Check sheet for the modelled part. Datum: model origin and axes. Units: mm. Face numbers are marked on the shaded views. A direction names the side the tool comes from. Give positions to 0.01 mm unless a question says otherwise; leave off trailing zeros. Loops run counter-clockwise (first coordinate to the right, second up) from the corner with the lowest first, then second, coordinate; pieces in that order, holes last. Notation, with made-up numbers: M -9,68 L 11,68 A29 ccw 11,102 Z; hole C -0.75,-36 d3. An arc over 180 degrees is marked long. Put each result on its own line as item: value. Start each with the question number.
```python
from build123d import *

# Parameters (mm, degrees)
CYLINDER019_R          = 2.5
CYLINDER019_DEPTH      = 10
CYLINDER016_R          = 2.5
CYLINDER016_DEPTH      = 10
CYLINDER017_W          = 35
CYLINDER017_H          = 19
CYLINDER017_ANGLE      = 25
CYLINDER018_W          = 35
CYLINDER018_H          = 19
CYLINDER018_ANGLE      = 25
BOX028_W               = 19
BOX028_H               = 50
BOX028_DEPTH           = 4
BOX003_W               = 140
BOX003_H               = 162
BOX003_DEPTH           = 4
BOX003_ROLL_ANGLE      = 25.000043
BOX003_PLACEMENT_ANGLE = 180
BOX032_W               = 19
BOX032_H               = 29
BOX032_DEPTH           = 8
BOX032_PLACEMENT_ANGLE = 25


with BuildPart() as m4s003:
    # Cylinder019 → Cylinder019 (new body)
    with BuildSketch(Plane(origin=(177.5, 240.5, 0), x_dir=(1, 0, 0), z_dir=(0, 0, 1))):
        Circle(CYLINDER019_R)
    extrude(amount=CYLINDER019_DEPTH)


with BuildPart() as m4lowcut001:
    # Cylinder016 → Cylinder016 (new body)
    with BuildSketch(Plane(origin=(177.5, 252.5, 0), x_dir=(1, 0, 0), z_dir=(0, 0, 1))):
        Circle(CYLINDER016_R)
    extrude(amount=CYLINDER016_DEPTH)

    # Fusion010: union m4s003
    add(m4s003.part)


with BuildPart() as cylinder017:
    # Cylinder017 → Cylinder017 (revolve)
    with BuildSketch(Plane(origin=(187, 283, 4), x_dir=(0, -1, 0), z_dir=(0, 0, -1))):
        with Locations((17.5, 9.5)):
            Rectangle(CYLINDER017_W, CYLINDER017_H)
    revolve(axis=Axis((187, 283, 4), (-1, 0, 0)), revolution_arc=CYLINDER017_ANGLE)


with BuildPart() as bottom002:
    # Cylinder018 → Cylinder018 (revolve)
    with BuildSketch(Plane(origin=(187, 292.5, 4), x_dir=(0, -1, 0), z_dir=(0, 0, -1))):
        with Locations((17.5, 9.5)):
            Rectangle(CYLINDER018_W, CYLINDER018_H)
    revolve(axis=Axis((187, 292.5, 4), (-1, 0, 0)), revolution_arc=CYLINDER018_ANGLE)

    # Cut016: cut Cylinder017
    add(cylinder017.part, mode=Mode.SUBTRACT)


with BuildPart() as bottomright:
    # Box028 → Box028 (new body)
    with BuildSketch(Plane(origin=(168, 233.5, 4), x_dir=(1, 0, 0), z_dir=(0, 0, 1))):
        with Locations((9.5, 25)):
            Rectangle(BOX028_W, BOX028_H)
    extrude(amount=BOX028_DEPTH)

    # Fusion009: union bottom002
    add(bottom002.part)

    # Cut017: cut m4lowCut001
    add(m4lowcut001.part, mode=Mode.SUBTRACT)


with BuildPart() as bottomright_1:
    # Cut017 placement: moved
    add(bottomright.part.moved(Location((144, 0, 0))))


with BuildPart() as solar_panel002:
    # Box003 → Box003 (new body)
    with BuildSketch(Plane.XY):
        with Locations((70, 81)):
            Rectangle(BOX003_W, BOX003_H)
    extrude(amount=BOX003_DEPTH)


with BuildPart() as solar_panel002_1:
    # Box003 roll: moved
    add(solar_panel002.part.rotate(Axis((0, 0, 0), (1, 0, 0)), BOX003_ROLL_ANGLE))


with BuildPart() as solar_panel002_2:
    # Box003 placement: moved
    add(solar_panel002_1.part.moved(Location((321.5, 284, 8))).rotate(Axis((321.5, 284, 8), (0, 0, 1)), BOX003_PLACEMENT_ANGLE))


with BuildPart() as topright001:
    # Box032 → Box032 (new body)
    with BuildSketch(Plane.XY):
        with Locations((9.5, 14.5)):
            Rectangle(BOX032_W, BOX032_H)
    extrude(amount=BOX032_DEPTH)


with BuildPart() as topright001_1:
    # Box032 placement: moved
    add(topright001.part.moved(Location((312, 260.906, 18.73))).rotate(Axis((312, 260.906, 18.73), (-1, 0, 0)), BOX032_PLACEMENT_ANGLE))

    # Cut024: cut solar Panel002
    add(solar_panel002_2.part, mode=Mode.SUBTRACT)

    # Fusion028: union bottomRight
    add(bottomright_1.part)


solid = topright001_1.part
```
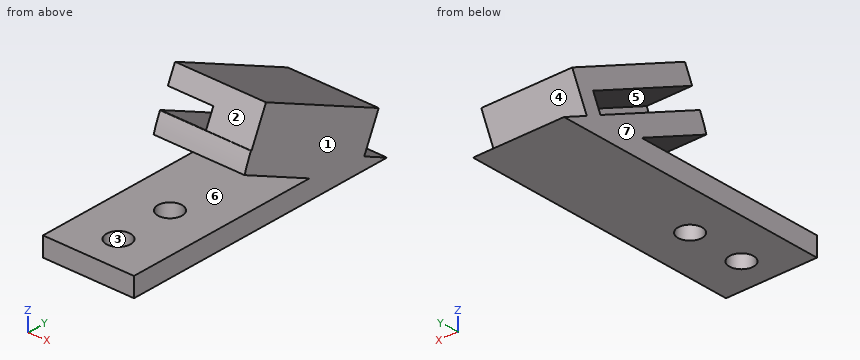
Q1. Access from +Z, -Z, +X, -X, +Y, -Y to the whole of each face (thin tool, end or side, straight path). Record for the marked faces 4, 5, 6 and 7.
Q2. Thickness scan on line 1 along X through (y, z) = (240.5, 5.35); line 2 along Z through (x, y) = (315.75, 268); line 3 along Z through (x, y) = (317, 271). Record the ranges inside material, lowest first. Write a range as [from, to].
Q3. Depth check by flat-ended pin: P1, Ø1.5, axis at x = 322.5, z = 16.5, coming from the -Y side; P2, Ø4, axis at x = 316, y = 247.5, coming from the +Z side; P3, Ø10, axis at x = 322, z = 20, coming from the -Y side. Enter the tip coordinate at first touch or a pass-through.
Q4. Mould release check, pull along X, two halves, no side actions. Record for the marked faces 1, 2 and 3: pulls with the +X half, pulls with the -X half, needs draft (parallel to the pull), parting line crosses it, or undercut.
Q5. Section check D-D, the plane z = 16.5. Record the cut outline in (x, y), then the cut area to 3 significant figures.
Q6. Section check B-B, the plane x = 319.75. Give the number of separate pieces and of enclosed holes in the cut face, then the cut area to 3 significant figures.
Q7. Section check A-A, the plane y = 240.5. Record the cut outline in (x, z), then the cut area to 3 significant figures.
Found:
1. face 4: +X, -X, +Y
1. face 5: -X
1. face 6: +X, -X, -Y
1. face 7: +Z, -Z, -X, +Y, -Y
2. line 1: x = [312, 319], [324, 331]
2. line 2: z = [4, 8], [10.99, 15.46], [19.87, 24.25]
2. line 3: z = [4, 8], [9.6, 14.06], [18.48, 22.85]
3. P1: stops at y = 259.53
3. P2: stops at z = 8
3. P3: stops at y = 259.29
4. face 1: pulls with the +X half
4. face 2: needs draft
4. face 3: undercut
5. outline: M 312,259.81 L 331,259.81 L 331,284.62 L 312,284.62 L 312,275.24 L 321.5,275.24 L 321.5,265.77 L 312,265.77 Z
5. area: 381 mm^2
6. separate pieces: 3
6. enclosed holes: 0
6. area: 405 mm^2
7. outline: M 312,4 L 319,4 L 319,8 L 312,8 Z; M 324,4 L 331,4 L 331,8 L 324,8 Z
7. area: 56.0 mm^2
